Autodesk Inventor part; units mm, degrees
ref_plane "YZ Plane" through (0, 0, 0) normal (1, 0, 0) x (0, 1, 0)
ref_plane "XZ Plane" through (0, 0, 0) normal (0, 1, 0) x (-1, 0, 0)
ref_plane "XY Plane" through (0, 0, 0) normal (0, 0, 1) x (1, 0, 0)
sketch "Sketch1" plane through (0, 0, 0) normal (0, 0, 1) x (1, 0, 0)
  circle A0 centre (0, 0) radius 52.07
  dimension "d0" = 104.14
extrude "Extrusion1" add sketch "Sketch1" along normal blind 7.62
ref_plane "Work Plane1" through (0, 0, 92.71) normal (0, 0, 1) x (1, 0, 0)
sketch "Sketch2" plane through (0, 0, 92.71) normal (0, 0, 1) x (1, 0, 0)
  circle A0 centre (0, 0) radius 52.07
  dimension "d4" = 104.14
extrude "Extrusion2" add sketch "Sketch2" along normal blind 7.62
sketch "Sketch3" plane through (0, 0, 7.62) normal (0, 0, 1) x (1, 0, 0)
  circle A0 centre (0, 0) radius 52.07
  line L0 (0, 52.07) -> (0, 41.91)
  line L1 (0, 41.91) -> (30.9004, 41.91)
  line L2 (0, 41.91) -> (-30.9004, 41.91)
  line L3 (0, 0) -> (20.3569, 0)
  dimension "d7" = 10.16
ref_plane "Work Plane2" through (0, 0, 7.62) normal (0, -1, 0) x (1, 0, 0)
extrude "Extrusion3" add sketch "Sketch3" along normal blind 87.5665 contours L1 L0 A0 | A0 L0 L2
mirror "Mirror1" about plane through (0, 0, 7.62) normal (0, -1, 0) of "Extrusion3"
sketch "Sketch4" plane through (0, 0, 100.33) normal (0, 0, 1) x (1, 0, 0)
  circle A0 centre (0, 0) radius 5.715
  dimension "d11" = 11.43
extrude "Extrusion4" cut sketch "Sketch4" against normal blind 101.6
sketch "Sketch5" plane through (0, 0, 7.62) normal (0, 0, 1) x (1, 0, 0)
  circle A0 centre (0, 0) radius 13.335
  circle A1 centre (0, 0) radius 5.715
  circle A2 centre (0, 0) radius 15.875
  dimension "d14" = 26.67
  dimension "d15" = 31.75
extrude "Extrusion5" add sketch "Sketch5" along normal blind 7.62 contours A2
sketch "Sketch6" plane through (-30.9004, -41.91, 92.71) normal (0, 1, 0) x (1, 0, 0)
  line L0 (61.8009, 85.09) -> (61.8009, 0)
  line L1 (61.8009, 42.545) -> (33.4028, 42.545)
  line L2 (0, 85.09) -> (0, 0)
  line L3 (0, 42.545) -> (61.8009, 42.545)
  line L4 (36.6154, -7.62) -> (25.1854, -7.62)
  line L5 (30.9004, -7.62) -> (30.9004, 92.71)
  circle A0 centre (30.9004, 42.545) radius 6.35
  point P0 (61.8009, 0)
  point P1 (58.0758, -2.4765)
  dimension "d53" = 12.7
extrude "Extrusion6" cut sketch "Sketch6" along normal mid plane 223.8375
sketch "Sketch10" plane through (0, 0, 0) normal (0, 0, -1) x (-1, 0, 0)
  circle A0 centre (0, 0) radius 5.715
  line L0 (5.715, 0) -> (12.065, 0)
  line L1 (12.065, 0) -> (12.065, 50.6529)
  circle A1 centre (0, 0) radius 52.07
  line L2 (12.065, 0) -> (12.065, -50.6529)
  line L3 (12.065, 0) -> (14.605, 0)
  line L4 (14.605, 0) -> (14.605, 49.9798)
  line L5 (14.605, 0) -> (14.605, -49.9798)
  line L6 (-5.715, 0) -> (-12.065, 0)
  line L7 (-12.065, 0) -> (-12.065, 50.6529)
  line L8 (-12.065, 0) -> (-12.065, -50.6529)
  line L9 (-12.065, 0) -> (-14.605, 0)
  line L10 (-14.605, 0) -> (-14.605, 49.9798)
  line L11 (-14.605, 0) -> (-14.605, -49.9798)
  dimension "d32" = 6.35
  dimension "d33" = 2.54
  dimension "d34" = 6.35
  dimension "d35" = 2.54
extrude "Extrusion10" add sketch "Sketch10" along normal blind 2.54 contours L3 L5 A1 L2 | L1 A1 L4 L3 | L9 L10 A1 L7 | L8 A1 L11 L9
sketch "Sketch14" plane through (0, 0, 0) normal (1, 0, 0) x (0, 1, 0)
  point P0 (0, 0)
sketch "Sketch15" plane through (-30.9004, -41.91, 7.62) normal (0, 1, 0) x (1, 0, 0)
  line L0 (61.8009, -85.09) -> (0, -85.09)
  line L1 (0, -85.09) -> (61.8009, -85.09)
  point P0 (30.9004, 7.62)
  point P1 (29.6304, -85.09)
ref_plane "Work Plane3" through (2.5024, -41.91, 50.165) normal (0, 1, 0) x (1, 0, 0)
sketch "Sketch18" plane through (-30.9004, -41.91, 7.62) normal (0, 1, 0) x (1, 0, 0)
  line L0 (61.8009, 0) -> (61.8009, -85.09)
  line L1 (61.8009, -42.545) -> (0, -42.545)
  line L2 (0, 0) -> (0, -85.09)
  line L3 (36.6154, -92.71) -> (25.1854, -92.71)
  line L4 (30.9004, -92.71) -> (30.9004, 7.62)
sketch "Sketch19" plane through (0, 0, 0) normal (1, 0, 0) x (0, 1, 0)
  line L0 (41.91, 7.62) -> (-41.91, 7.62)
  line L1 (27.4323, 7.62) -> (27.4323, 20.239)
  line L2 (27.4323, 20.239) -> (-18.8978, 20.239)
  line L3 (-18.8978, 20.239) -> (-18.8978, 7.62)
  line L4 (27.4323, 7.62) -> (-18.8978, 7.62)
  point P0 (0, 0)
extrude "Extrusion16" cut sketch "Sketch19" along normal mid plane 101.6
sketch "Sketch20" plane through (-30.9004, 41.91, 7.62) normal (0, -1, 0) x (1, 0, 0)
  line L0 (0, 0) -> (0, 85.09)
  line L1 (0, 42.545) -> (61.8009, 42.545)
  line L2 (61.8009, 0) -> (61.8009, 85.09)
  circle A0 centre (30.9004, 42.545) radius 16.51
  circle A1 centre (30.9004, 42.545) radius 19.05
  point P0 (30.9004, -7.62)
  dimension "d61" = 33.02
  dimension "d62" = 38.1
extrude "Extrusion17" add sketch "Sketch20" along normal blind 7.62 contours A0 L1 A1 | L1 A1 A0
mirror "Mirror3" about plane through (0, 0, 7.62) normal (0, -1, 0) of "Extrusion17"
sketch "Sketch21" plane through (-30.9004, -41.91, 92.71) normal (0, 1, 0) x (1, 0, 0)
  line L0 (0, 85.09) -> (61.8009, 85.09)
  line L1 (30.9004, 85.09) -> (32.1704, 85.09)
  line L2 (32.1704, 85.09) -> (30.9004, 85.09)
  line L3 (30.9004, 85.09) -> (29.6304, 85.09)
  line L4 (29.6304, 85.09) -> (29.6304, 61.5526)
  circle A0 centre (30.9004, 42.545) radius 19.05
  line L5 (32.1704, 85.09) -> (32.1704, 61.5526)
  line L6 (29.6304, 61.5526) -> (32.1704, 61.5526)
  line L7 (61.8009, 0) -> (0, 0)
  line L8 (30.9004, 0) -> (29.6304, 0)
  line L9 (29.6304, 0) -> (32.1704, 0)
  line L10 (32.1704, 0) -> (32.1704, 23.5374)
  line L11 (29.6304, 0) -> (29.6304, 23.5374)
  line L12 (32.1704, 23.5374) -> (29.6304, 23.5374)
  point P0 (30.9004, 92.71)
  dimension "d65" = 1.27
  dimension "d66" = 1.27
  dimension "d67" = 1.27
  dimension "d68" = 1.27
  dimension "d69" = 2.54
extrude "Extrusion18" add sketch "Sketch21" along normal blind 2.54 contours L0 L5 A0 L4 | A0 L10 L7 L11
mirror "Mirror4" about plane through (0, 0, 7.62) normal (0, -1, 0) of "Extrusion18"
properties part number "Fourth Diff"
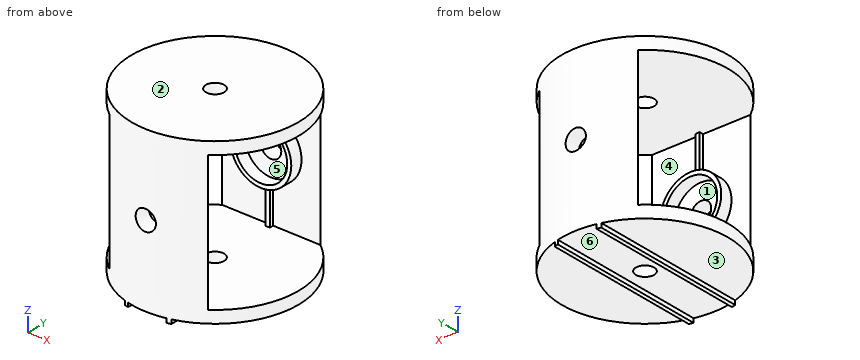
For this review, take the finished solid that the model builds, in its own axes (mm). Face numbers are marked on the shaded views. A direction names the side the tool comes from. Give positions to 0.01 mm unless a question says otherwise; leave off trailing zeros. Write each loop counter-clockwise with the first axis right and the second up, starting at its lowest first coordinate (ties: lowest second). Pieces come first, ordered by that corner, then holes. Notation, with made-up numbers: M -13,77 L 35,77 A23 cw 35,90 Z; hole C 19,25.5 d4. An arc over 180 degrees is marked long. One line per item, written item: value.
1) Take a section at B-B, the plane y = 0. Write out the cut boundary in (x, z) (3 decimals), then the cut area to 3 significant figures.
Results are:
outline: M -52.07,0 L -14.605,0 L -14.605,-2.54 L -12.065,-2.54 L -12.065,0 L -5.715,0 L -5.715,7.62 L -52.07,7.62 Z; M -52.07,92.71 L -5.715,92.71 L -5.715,100.33 L -52.07,100.33 Z; M 5.715,0 L 12.065,0 L 12.065,-2.54 L 14.605,-2.54 L 14.605,0 L 52.07,0 L 52.07,7.62 L 5.715,7.62 Z; M 5.715,92.71 L 52.07,92.71 L 52.07,100.33 L 5.715,100.33 Z
area: 1,430 mm²
2) For P1, Ø1, axis at x = 12, z = 52.5, coming from the -Y side; P2, Ø0.8, axis at y = 4.5, z = -1.5, coming from the -X side (3 decimals); P3, Ø12, axis at x = 1, y = 13.5, coming from the -Z side; P4, Ø19, axis at x = 5, z = 42, coming from the +Y side, all flat-tipped, find the tip position at first contact; note any pin that passes through.
Results are:
P1: stops at y = -50.78
P2: stops at x = -14.605
P3: stops at z = 0
P4: stops at y = 52.07
3) The part is to be moulded in two halves that separate along Z. For the marked faces 1, 2 and 3, say which applies: +Z half, -Z half, draft (parallel to the pull), parting line (faces both ways), or undercut.
Results are:
face 1: undercut
face 2: +Z half
face 3: -Z half
4) Take a section at D-D, the plane y = 15.5. Write out the cut boundary in (x, z) (1 decimal).
Results are:
outline: M -49.7,0 L -14.6,0 L -14.6,-2.5 L -12.1,-2.5 L -12.1,0 L 12.1,0 L 12.1,-2.5 L 14.6,-2.5 L 14.6,0 L 49.7,0 L 49.7,7.6 L -49.7,7.6 Z; M -49.7,92.7 L 49.7,92.7 L 49.7,100.3 L -49.7,100.3 Z
5) For the marked faces 4, 5 and 6, list the 3-axis set-ups (+Z, -Z, +X, -X, +Y, -Y) from which the entire face can be reached by the end or side of a thin tool; tool diameter is ignored.
Results are:
face 4: +X
face 5: none
face 6: -Z, +Y, -Y
6) Take a section at C-C, the plane x = -36.5. Write out the cut boundary in (y, z).
Results are:
outline: M -37.14,0 L 37.14,0 L 37.14,7.62 L -37.14,7.62 Z; M -37.14,92.71 L 37.14,92.71 L 37.14,100.33 L -37.14,100.33 Z
7) For line 1 (Z direction, x = 0, y = -36.5) (3 decimals); line 2 (Y direction, x = 0, z = 5) (3 decimals); line 3 (Z direction, x = -41.5, y = 14.5), list the stretches that pass through material, from the lowest coordinate up. Write a range as from..to.
Results are:
line 1: z = 0..7.62, 31.115..33.655, 66.675..69.215, 92.71..100.33
line 2: y = -52.07..-5.715, 5.715..52.07
line 3: z = 0..7.62, 92.71..100.33
8) Take a section at A-A, the plane z = 24. Write out the cut boundary in (x, y), then the cut area to 3 significant figures.
Results are:
outline: M -30.9,-41.91 A52.07 ccw 30.9,-41.91 L 1.27,-41.91 L 1.27,-39.37 L -1.27,-39.37 L -1.27,-41.91 Z; M -30.9,41.91 L -1.27,41.91 L -1.27,39.37 L 1.27,39.37 L 1.27,41.91 L 30.9,41.91 A52.07 ccw Z
area: 868 mm²
